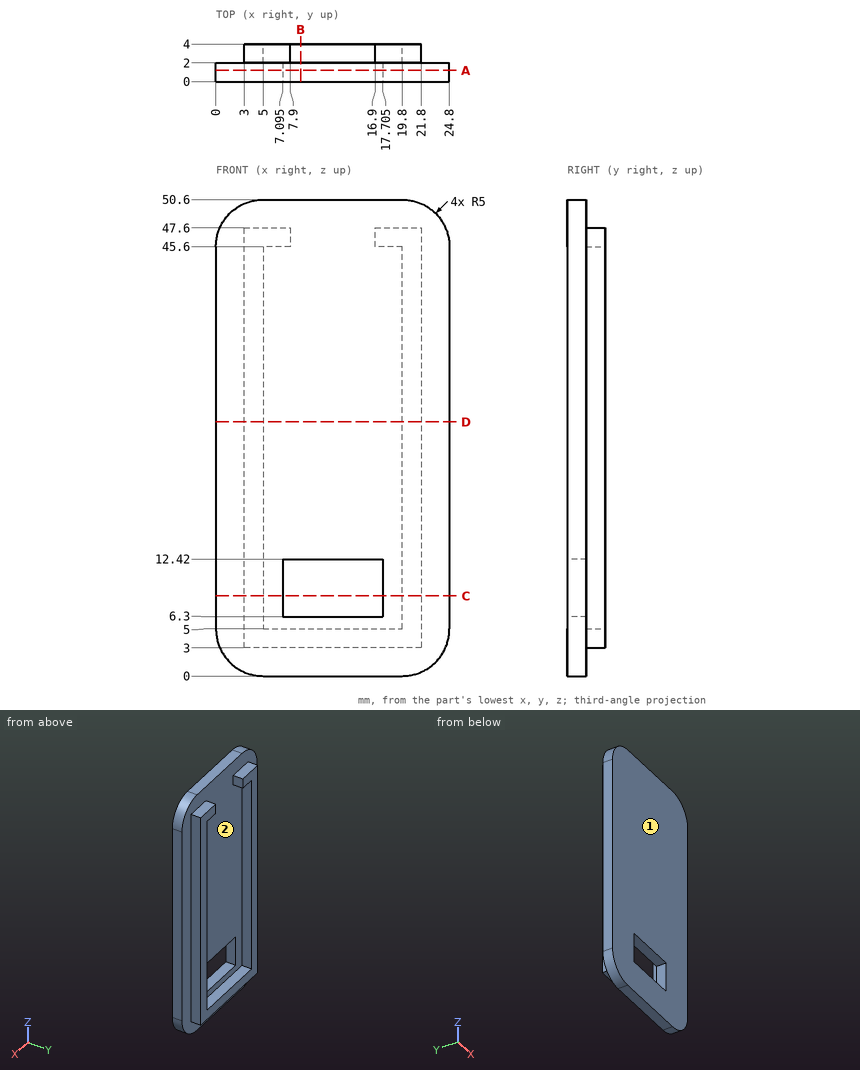
Source: three-view drawing plus pictorial views. Frame: mm from the lowest corner of the part. Give positions to 0.01 mm unless a question says otherwise; leave off trailing zeros. Write each loop counter-clockwise with the first axis right and the second up, starting at its lowest first coordinate (ties: lowest second). Pieces come first, ordered by that corner, then holes. Notation, with made-up numbers: M -22.75,-11.75 L 30.25,-11.75 A18 ccw 30.25,17.25 Z; hole C 67,12.5 d7. An arc over 180 degrees is marked long. Use one line per item in the form item = value.
1. Cut plane D-D on z = 27. Return loops of the section in (x, y).
Outcome:
outline = M 0,0 L 24.8,0 L 24.8,2 L 21.8,2 L 21.8,4 L 19.8,4 L 19.8,2 L 5,2 L 5,4 L 3,4 L 3,2 L 0,2 Z
2. Cut plane C-C on z = 8.5. Return loops of the section in (x, y) (3 decimals).
Outcome:
outline = M 0,0 L 7.095,0 L 7.095,2 L 5,2 L 5,4 L 3,4 L 3,2 L 0,2 Z; M 17.705,0 L 24.8,0 L 24.8,2 L 21.8,2 L 21.8,4 L 19.8,4 L 19.8,2 L 17.705,2 Z
3. First-contact query: P1, Ø0.6, axis at y = 3, z = 47, coming from the +X side; P2, Ø0.6, axis at x = 14, y = 3, coming from the +Z side; P3, Ø1.6, axis at x = 6, y = 3, coming from the -Z side. Flat tips, straight axial feed; report the tip coordinate or a pass-through.
Outcome:
P1 = 21.8
P2 = 5
P3 = 3
4. Mould query, pull axis Z, two halves, no side actions, for the marked faces 1 and 2. Classes: released by +Z, released by -Z, zero draft, split by the parting line, or undercut.
Outcome:
face_1 = zero draft
face_2 = undercut
5. Cut plane A-A on y = 1.2. Return loops of the section in (x, z) (3 decimals), and give its area (3 significant figures).
Outcome:
outline = M 0,5 A5 ccw 5,0 L 19.8,0 A5 ccw 24.8,5 L 24.8,45.6 A5 ccw 19.8,50.6 L 5,50.6 A5 ccw 0,45.6 Z; hole M 7.095,6.3 L 17.705,6.3 L 17.705,12.42 L 7.095,12.42 Z
area = 1,170 mm²
6. Ray query, L1, parallel to X at y = 3, z = 26; L2, parallel to Z at x = 7.5, y = 1.6; L3, parallel to Z at x = 16.75, y = 2.75. Return the intervals inside material, ascending.
Outcome:
L1 = 3 to 5, 19.8 to 21.8
L2 = 0 to 6.3, 12.42 to 50.6
L3 = 3 to 5
7. Cut plane B-B on x = 9. Return loops of the section in (y, z).
Outcome:
outline = M 0,0 L 2,0 L 2,3 L 4,3 L 4,5 L 2,5 L 2,6.3 L 0,6.3 Z; M 0,12.42 L 2,12.42 L 2,50.6 L 0,50.6 Z
